from build123d import *

# Parameters (mm, degrees)
SKETCH4_W            = 52
SKETCH4_H            = 80
BOSS_EXTRUDE4_DEPTH  = 5
SKETCH6_W            = 5
SKETCH6_H            = 80
BOSS_EXTRUDE5_DEPTH  = 35
SKETCH7_W            = 5
SKETCH7_H            = 80
BOSS_EXTRUDE6_DEPTH  = 35
SKETCH8_W            = 42
SKETCH8_H            = 5
BOSS_EXTRUDE7_DEPTH  = 5
FILLET2_R            = 3
FILLET3_R            = 3
FILLET4_R            = 3
SKETCH9_R            = 8
SKETCH9_R_2          = 5
CUT_EXTRUDE1_DEPTH   = 5
SKETCH10_W           = 5
SKETCH10_H           = 2
BOSS_EXTRUDE8_DEPTH  = 1
SKETCH11_W           = 40
SKETCH11_H           = 80
BOSS_EXTRUDE9_DEPTH  = 5
SKETCH12_W           = 40
SKETCH12_H           = 5
BOSS_EXTRUDE11_DEPTH = 30
FILLET6_R            = 3
SKETCH13_W           = 10.232646845
SKETCH13_H           = 7.639513139
SKETCH13_W_2         = 10.199522787
SKETCH13_H_2         = 7.142143056
CUT_EXTRUDE2_DEPTH   = 30


with BuildPart() as part:
    # Sketch4 → Boss-Extrude4 (new body)
    with BuildSketch(Plane(origin=(0, 0, 0), x_dir=(1, 0, 0), z_dir=(0, 1, 0))):
        with Locations((26, 40)):
            Rectangle(SKETCH4_W, SKETCH4_H)
    extrude(amount=BOSS_EXTRUDE4_DEPTH)

    # Sketch6 → Boss-Extrude5 (add)
    with BuildSketch(Plane.XZ):
        with Locations((49.5, -40)):
            Rectangle(SKETCH6_W, SKETCH6_H)
    extrude(amount=-BOSS_EXTRUDE5_DEPTH)

    # Sketch7 → Boss-Extrude6 (add)
    with BuildSketch(Plane(origin=(0, 0, 0), x_dir=(-1, 0, 0), z_dir=(0, -1, 0))):
        with Locations((-2.5, 40)):
            Rectangle(SKETCH7_W, SKETCH7_H)
    extrude(amount=-BOSS_EXTRUDE6_DEPTH)

    # Sketch8 → Boss-Extrude7 (add)
    with BuildSketch(Plane(origin=(0, 5, 0), x_dir=(1, 0, 0), z_dir=(0, 1, 0))):
        with Locations((26, 72.5)):
            Rectangle(SKETCH8_W, SKETCH8_H)
        with Locations((26, 7.5)):
            Rectangle(SKETCH8_W, SKETCH8_H)
    extrude(amount=BOSS_EXTRUDE7_DEPTH)

    # Fillet2
    fillet2_edges = [part.edges().sort_by_distance(p)[0] for p in [
        (52, 0, -40),
    ]]
    fillet(fillet2_edges, radius=FILLET2_R)

    # Fillet3
    fillet3_edges = [part.edges().sort_by_distance(p)[0] for p in [
        (47, 5, -2.5),
    ]]
    fillet(fillet3_edges, radius=FILLET3_R)

    # Fillet4
    fillet4_edges = [part.edges().sort_by_distance(p)[0] for p in [
        (5, 5, -77.5),
        (5, 5, -40),
        (47, 5, -77.5),
        (0, 0, -40),
        (5, 5, -2.5),
        (47, 5, -40),
    ]]
    fillet(fillet4_edges, radius=FILLET4_R)

    # Sketch9 → Cut-Extrude1 (cut)
    with BuildSketch(Plane(origin=(52, 0, 0), x_dir=(0, 0, -1), z_dir=(1, 0, 0))):
        with Locations((20, 19)):
            Circle(SKETCH9_R)
        with Locations((40, 19)):
            Circle(SKETCH9_R)
        with Locations((65, 19)):
            Circle(SKETCH9_R_2)
    extrude(amount=-CUT_EXTRUDE1_DEPTH, mode=Mode.SUBTRACT)

    # Sketch10 → Boss-Extrude8 (add)
    with BuildSketch(Plane(origin=(0, 0, 0), x_dir=(1, 0, 0), z_dir=(0, 1, 0))):
        with Locations((0.5, 1)):
            Rectangle(SKETCH10_W, SKETCH10_H)
        with Locations((0.5, 79)):
            Rectangle(SKETCH10_W, SKETCH10_H)
    extrude(amount=BOSS_EXTRUDE8_DEPTH)

    # Sketch11 → Boss-Extrude9 (add)
    with BuildSketch(Plane.XZ):
        with Locations((-22, -40)):
            Rectangle(SKETCH11_W, SKETCH11_H)
    extrude(amount=-BOSS_EXTRUDE9_DEPTH)

    # Sketch12 → Boss-Extrude11 (add)
    with BuildSketch(Plane.XZ):
        with Locations((-22, -2.5)):
            Rectangle(SKETCH12_W, SKETCH12_H)
        with Locations((-22, -77.5)):
            Rectangle(SKETCH12_W, SKETCH12_H)
    extrude(amount=-BOSS_EXTRUDE11_DEPTH)

    # Fillet6
    fillet6_edges = [part.edges().sort_by_distance(p)[0] for p in [
        (-42, 30, -2.5),
        (-2, 30, -2.5),
        (-42, 30, -77.5),
        (-2, 30, -77.5),
    ]]
    fillet(fillet6_edges, radius=FILLET6_R)

    # Sketch13 → Cut-Extrude2 (cut)
    with BuildSketch(Plane(origin=(5, 0, 0), x_dir=(0, 0, -1), z_dir=(1, 0, 0))):
        with Locations((14.052030706, 21.139780505)):
            Rectangle(SKETCH13_W, SKETCH13_H)
        with Locations((59.580586702, 21.388465546)):
            Rectangle(SKETCH13_W_2, SKETCH13_H_2)
    extrude(amount=-CUT_EXTRUDE2_DEPTH, mode=Mode.SUBTRACT)


solid = part.part
CAD build for the part. Positions are in the model's coordinates, mm. A direction names the side the tool comes from. Round coordinates to 2 decimals unless told otherwise and drop trailing zeros. Write each loop counter-clockwise with the first axis right and the second up, starting at its lowest first coordinate (ties: lowest second). Pieces come first, ordered by that corner, then holes. Notation, with made-up numbers: M -18.75,73.5 L 13.25,73.5 A12 ccw 13.25,94.5 Z; hole C -32,14 d2. An arc over 180 degrees is marked long. Use a Markdown table: item, result. Add a question column.
1. Drill centre lines: probe 1 along X at (y, z) = (12, -32.5); probe 2 along Z at (x, y) = (4.5, 23); probe 3 along Z at (x, y) = (-18, 20.5). Where is each one in solid material? Low to high.
2. Slice it at D-D on y = 32. Give the cut face in (x, z).
3. 3-axis set-ups, long thin cutter, end or side, ignore diameter. For faces 4 (the face through (26, 7, -70)), 5 (the face through (26, 7, -5)), 6 (the face through (50, 19, -12)), 7 (the face through (3, 24.96, -14)): which of +Z, -Z, +X, -X, +Y, -Y reach the whole face in a straight line?
4. Pull direction Y, two halves, no side cores. Call faces 1 (the face through (3, 21, -19.168)), 2 (the face through (-42, 4, -40)), 3 (the face through (46.14, 5.9, -77.54)): released by +Y, released by -Y, zero draft, split by the parting line, or undercut.
5. Slice it at C-C on x = -24. Give the cut face in (y, z).
6. Slice it at B-B on z = -40. Give the cut face in (x, y), then the cut area to 3 significant figures.
7. Flat gauge pins, fed straight in: P1, Ø5, axis at y = 15, z = -16.5, coming from the +X side; P2, Ø4, axis at x = -29.5, z = -1.5, coming from the +Y side; P3, Ø1.5, axis at x = 33, y = 8.5, coming from the +Z side. Where does each tip first touch, or does it go through?
8. Slice it at A-A on y = 16. Give the cut face in (x, z).
Reply:
| question | item | result |
|---|---|---|
| 1 | probe 1 | x = 0 to 5, 47 to 52 |
| 1 | probe 2 | z = -80 to -64.68, -54.48 to -19.17, -8.94 to 0 |
| 1 | probe 3 | z = -80 to -75, -5 to 0 |
| 2 | outline | M 0,-80 L 5,-80 L 5,0 L 0,0 Z; M 47,-80 L 52,-80 L 52,0 L 47,0 Z |
| 3 | face 4 | +Y |
| 3 | face 5 | +Z, +Y |
| 3 | face 6 | +X |
| 3 | face 7 | -X |
| 4 | face 1 | undercut |
| 4 | face 2 | zero draft |
| 4 | face 3 | released by +Y |
| 5 | outline | M 0,-80 L 30,-80 L 30,-75 L 5,-75 L 5,-5 L 30,-5 L 30,0 L 0,0 Z |
| 6 | outline | M -42,0 L -2,0 L -2,5 L -42,5 Z; M 0,3 A3 ccw 3,0 L 49,0 A3 ccw 52,3 L 52,11 L 47,11 L 47,8 A3 cw 44,5 L 8,5 A3 cw 5,8 L 5,35 L 0,35 Z; M 47,27 L 52,27 L 52,35 L 47,35 Z |
| 6 | area | 680 mm^2 |
| 7 | P1 | stops at x = 5 |
| 7 | P2 | stops at y = 30 |
| 7 | P3 | stops at z = -5 |
| 8 | outline | M -42,-80 L -2,-80 L -2,-75 L -42,-75 Z; M -42,-5 L -2,-5 L -2,0 L -42,0 Z; M 0,-80 L 5,-80 L 5,0 L 0,0 Z; M 47,-80 L 52,-80 L 52,-69 L 47,-69 Z; M 47,-61 L 52,-61 L 52,-47.42 L 47,-47.42 Z; M 47,-32.58 L 52,-32.58 L 52,-27.42 L 47,-27.42 Z; M 47,-12.58 L 52,-12.58 L 52,0 L 47,0 Z |
